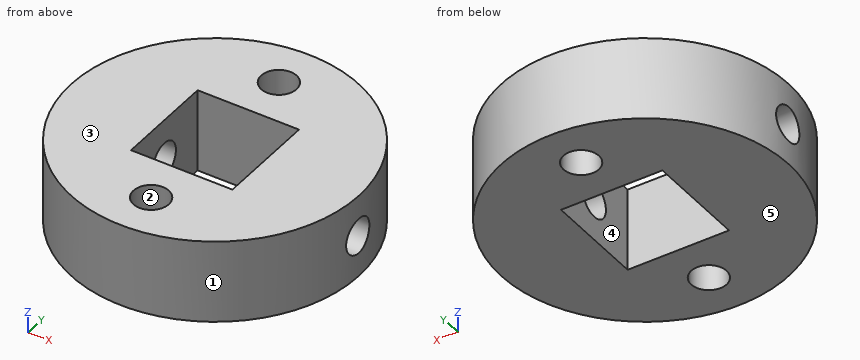
```python
from build123d import *

# Parameters (mm, degrees)
SKETCH1_R                           = 10.9855
SKETCH1_W                           = 7.747
SKETCH1_H                           = 7.747
BOSS_EXTRUDE1_DEPTH                 = 6.35
F_6_32_TAPPED_HOLE1_D               = 2.7051
F_6_32_TAPPED_HOLE1_DEPTH           = 7.112
F_6_32_TAPPED_HOLE1_ON_FACE_2_D     = 2.7051
F_6_32_TAPPED_HOLE1_ON_FACE_2_DEPTH = 7.112
F_6_32_TAPPED_HOLE2_D               = 2.7051
F_6_32_TAPPED_HOLE4_D               = 2.7051


with BuildPart() as part:
    # Sketch1 → Boss-Extrude1 (new body)
    with BuildSketch(Plane.XY):
        Circle(SKETCH1_R)
        Rectangle(SKETCH1_W, SKETCH1_H, mode=Mode.SUBTRACT)
    extrude(amount=BOSS_EXTRUDE1_DEPTH)

    # #6-32 Tapped Hole1
    with Locations(Plane(origin=(10.9855, 0, 3.175), x_dir=(0, 0, 1), z_dir=(1, 0, 0))):
        with Locations((0, 0)):
            Hole(F_6_32_TAPPED_HOLE1_D / 2, depth=F_6_32_TAPPED_HOLE1_DEPTH)

    # #6-32 Tapped Hole1 on face 2
    with Locations(Plane(origin=(3.8735, 0, 3.175), x_dir=(0, 0, -1), z_dir=(-1, 0, 0))):
        with Locations((0, 0)):
            Hole(F_6_32_TAPPED_HOLE1_ON_FACE_2_D / 2, depth=F_6_32_TAPPED_HOLE1_ON_FACE_2_DEPTH)

    # #6-32 Tapped Hole2 (through all)
    with Locations(Plane(origin=(-3.8735, 0, 0), x_dir=(0, 0, -1), z_dir=(1, 0, 0))):
        with Locations((-3.175, 0)):
            Hole(F_6_32_TAPPED_HOLE2_D / 2)

    # #6-32 Tapped Hole4 (through all)
    with Locations(Plane(origin=(0, 0, 0), x_dir=(-1, 0, 0), z_dir=(0, 0, -1))):
        with Locations((0, -7.4295), (0, 7.4295)):
            Hole(F_6_32_TAPPED_HOLE4_D / 2)


solid = part.part
```
Here's how the part is built. I have some questions about the finished solid (model axes, mm). Face numbers are marked on the shaded views. A direction names the side the tool comes from. Round coordinates to 2 decimals unless told otherwise and drop trailing zeros. Loops run counter-clockwise (first coordinate to the right, second up) from the corner with the lowest first, then second, coordinate; pieces in that order, holes last.
1. Suppose I cut it at D-D, the plane x = -3.25. Please give me the cut outline in (y, z), and give its area (3 significant figures).
Answers:
outline: (-10.49, 0) - (-3.87, 0) - (-3.87, 6.35) - (-10.49, 6.35) - close; (3.87, 0) - (10.49, 0) - (10.49, 6.35) - (3.87, 6.35) - close
area: 84.1 mm2
2. Will these pins go through, and if not, where does the flat tip stop? pin 1 (1.9 mm diameter, centred on x = 1.5, z = 1.5, fed in from +Y); pin 2 (1.9 mm diameter, centred on y = 1, z = 3, fed in from +X); pin 3 (1.5 mm diameter, centred on y = 8.5, z = 4, fed in from +X); pin 4 (1.6 mm diameter, centred on x = 0, y = 7.43, fed in from +Z).
Answers:
pin 1: stops at y = 10.97
pin 2: stops at x = 10.96
pin 3: stops at x = 7.79
pin 4: passes through
3. Suppose I cut it at C-C, the plane x = 0. Please give me the cut outline in (y, z), and give its area (3 significant figures).
Answers:
outline: (-10.99, 0) - (-8.78, 0) - (-8.78, 6.35) - (-10.99, 6.35) - close; (-6.08, 0) - (-3.87, 0) - (-3.87, 6.35) - (-6.08, 6.35) - close; (3.87, 0) - (6.08, 0) - (6.08, 6.35) - (3.87, 6.35) - close; (8.78, 0) - (10.99, 0) - (10.99, 6.35) - (8.78, 6.35) - close
area: 56.0 mm2
4. If I drill on probe 1 along Y at (x, z) = (0, 3.75); probe 2 along Z at (x, y) = (-8.5, 0); probe 3 along X at (y, z) = (-8.5, 1), over which ranges is the centre line in solid material (lowest first)?
Answers:
probe 1: y = -10.99 to -8.78, -6.08 to -3.87, 3.87 to 6.08, 8.78 to 10.99
probe 2: z = 0 to 1.82, 4.53 to 6.35
probe 3: x = -6.96 to -0.83, 0.83 to 6.96
5. For the marked faces 4 and 5, which set-ups out of +Z, -Z, +X, -X, +Y, -Y let a thin tool reach every point of the face, with its end or its side?
Answers:
face 4: +Z, -Z
face 5: -Z, +X, -X, +Y, -Y
6. Thinking about a two-plate mould opening in X: for the marked faces 1, 2 and 3, which applies, released by +X, released by -X, zero draft, split by the parting line, or undercut?
Answers:
face 1: split by the parting line
face 2: undercut
face 3: zero draft
7. Suppose I cut it at A-A, the plane z = 3.5. Please give me the cut outline in (x, y), and give its area (3 significant figures).
Answers:
outline: (-10.91, -1.31) arc R10.99 ccw to (10.91, -1.31) - (3.87, -1.31) - (3.87, -3.87) - (-3.87, -3.87) - (-3.87, -1.31) - close; (-10.91, 1.31) - (-3.87, 1.31) - (-3.87, 3.87) - (3.87, 3.87) - (3.87, 1.31) - (10.91, 1.31) arc R10.99 ccw to start; hole circle Ø2.71 at (0, -7.43); hole circle Ø2.71 at (0, 7.43)
area: 270 mm2
8. Suppose I cut it at B-B, the plane y = 0. Please give me the cut outline in (x, z), and give its area (3 significant figures).
Answers:
outline: (-10.99, 0) - (-3.87, 0) - (-3.87, 1.82) - (-10.99, 1.82) - close; (-10.99, 4.53) - (-3.87, 4.53) - (-3.87, 6.35) - (-10.99, 6.35) - close; (3.87, 0) - (10.99, 0) - (10.99, 1.82) - (3.87, 1.82) - close; (3.87, 4.53) - (10.99, 4.53) - (10.99, 6.35) - (3.87, 6.35) - close
area: 51.8 mm2
